Check sheet for the drawn part. Datum: minimum x, y, z corner. Units: mm. Give positions to 0.01 mm unless a question says otherwise; leave off trailing zeros. Order: outer loops, then holes, each group sorted by start corner. A loop starts at its lowest first (then second) coordinate and runs counter-clockwise, first axis right, second up.
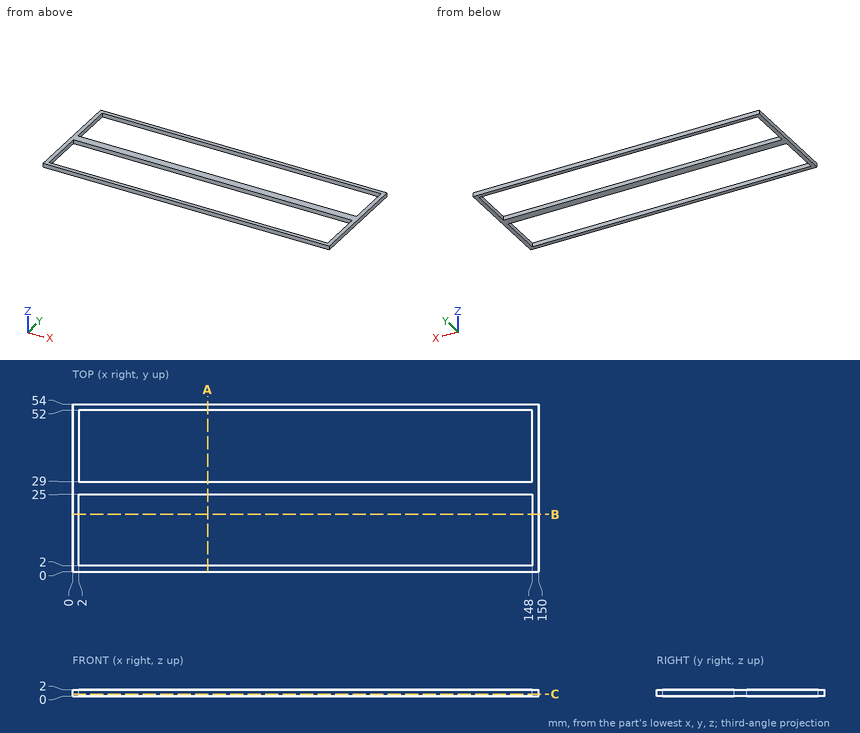
(1) Section check B-B, the plane y = 18.5. Enter the section's corners in (x, z), then the cut area to 3 significant figures.
Solved:
outline: (0, 0) - (2, 0) - (2, 2) - (0, 2) - close; (148, 0) - (150, 0) - (150, 2) - (148, 2) - close
area: 8.00 mm2
(2) Section check A-A, the plane x = 43.5. Enter the section's corners in (y, z), then the cut area to 3 significant figures.
Solved:
outline: (0, 0) - (2, 0) - (2, 2) - (0, 2) - close; (25, 0) - (29, 0) - (29, 2) - (25, 2) - close; (52, 0) - (54, 0) - (54, 2) - (52, 2) - close
area: 16.0 mm2
(3) Scan lines: line 1 (Y direction, x = 16, z = 1.2); line 2 (X direction, y = 3.5, z = 0.3). Record each from-to range of solid material in increasing order.
Solved:
line 1: y = 0 to 2, 25 to 29, 52 to 54
line 2: x = 0 to 2, 148 to 150
(4) Section check C-C, the plane z = 0.6. Enter the section's corners in (x, y).
Solved:
outline: (0, 0) - (150, 0) - (150, 54) - (0, 54) - close; hole (2, 2) - (148, 2) - (148, 25) - (2, 25) - close; hole (2, 29) - (148, 29) - (148, 52) - (2, 52) - close
